Study the drawing (mm; zero at the part's minimum x, y, z) and answer. A direction names the side the tool comes from. Give positions to 0.01 mm unless a question says otherwise; leave off trailing zeros. Order: outer loops, then holes, each group sorted by start corner. A loop starts at its lowest first (then second) coordinate and runs counter-clockwise, first axis right, second up. Notation, with made-up numbers: (-12.5, -14.5) - (41.5, -14.5) arc R15 ccw to (41.5, -4.5) - close; hole circle Ø4 at (70.5, -37.5). An arc over 180 degrees is marked (long way). Write each question's results on one line, items separated by ' | '. Start each with the question number.
1. Which of the six approach directions +Z, -Z, +X, -X, +Y, -Y give full straight-line access (tool end or side, diameter ignored) to the marked faces 1, 2 and 3?
2. Section B-B (x = 14.6) is taken. Give the vertices of the cut face in (y, z).
3. Determine the mould class of the marked faces 4, 5, 6 and 7 for opening direction X: released by +X, released by -X, zero draft, split by the parting line, or undercut.
4. Flat-ended cylindrical pins translate along their axes: pin 1 (5 mm diameter, centred on x = 3.5, z = 3, fed in from -Y); pin 2 (2 mm diameter, centred on x = 5, y = 1.5, fed in from +Z); pin 3 (0.6 mm diameter, centred on y = 1.5, z = 3, fed in from -X). Find the tip coordinate at first contact, or state that the pin passes through.
5. Section A-A (z = 7) is taken. Give the vertices of the cut face in (x, y), and give its area (3 significant figures).
6. Section D-D (x = 2) is taken. Give the vertices of the cut face in (y, z), and give its area (3 significant figures).
7. Find the intervals of material crossed by L1, parallel to X at y = 5.05, z = 8; L2, parallel to Z at x = 2, y = 5.65; L3, parallel to Z at x = 14.6, y = 1.6, in increasing order.
8. Section C-C (z = 8) is taken. Give the vertices of the cut face in (x, y), and give its area (3 significant figures).
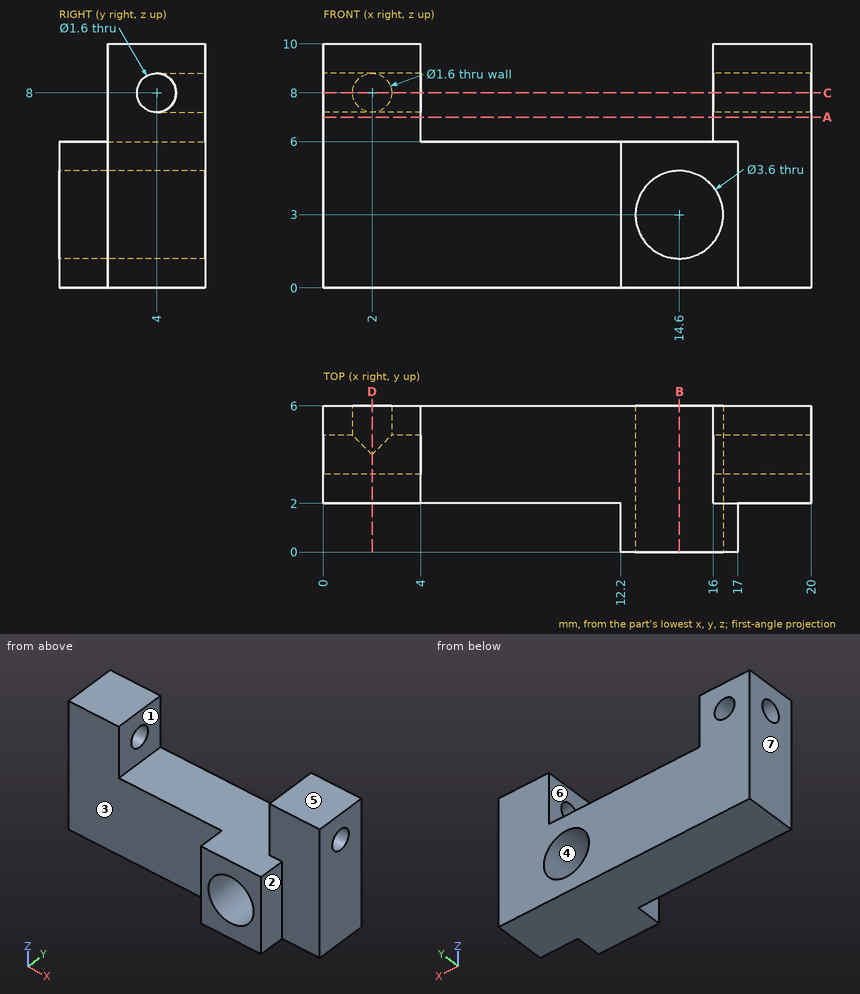
Reported:
1) face 1: +Z, +Y, -Y | face 2: +Z, -Z, +X, -Y | face 3: +Z, -Z, -X, -Y
2) outline: (0, 0) - (6, 0) - (6, 1.2) - (0, 1.2) - close; (0, 4.8) - (6, 4.8) - (6, 6) - (0, 6) - close
3) face 4: undercut | face 5: zero draft | face 6: undercut | face 7: released by -X
4) pin 1: y = 2 | pin 2: z = 6 | pin 3: x = 12.2
5) outline: (0, 2) - (4, 2) - (4, 6) - (0, 6) - close; (16, 2) - (20, 2) - (20, 6) - (16, 6) - close | area: 32.0 mm²
6) outline: (2, 0) - (6, 0) - (6, 7.2) - (4, 7.2) arc R0.8 cw to (4, 8.8) - (6, 8.8) - (6, 10) - (2, 10) - close | area: 35.8 mm²
7) L1: 0 to 1.2, 2.8 to 4, 16 to 20 | L2: 0 to 7.2, 8.8 to 10 | L3: 0 to 1.2, 4.8 to 6
8) outline: (0, 2) - (4, 2) - (4, 3.2) - (0, 3.2) - close; (0, 4.8) - (1.2, 4.8) - (1.2, 6) - (0, 6) - close; (2.8, 4.8) - (4, 4.8) - (4, 6) - (2.8, 6) - close; (16, 2) - (20, 2) - (20, 3.2) - (16, 3.2) - close; (16, 4.8) - (20, 4.8) - (20, 6) - (16, 6) - close | area: 17.3 mm²
